Verification items for the finished model (mm, model axes). A direction names the side the tool comes from. Give positions to 0.01 mm unless a question says otherwise; leave off trailing zeros. Loops run counter-clockwise (first coordinate to the right, second up) from the corner with the lowest first, then second, coordinate; pieces in that order, holes last. Notation, with made-up numbers: (-2.5, 42) - (7.5, 42) arc R26 cw to (7.5, 61) - close; hole circle Ø10 at (48.5, -32.75). An arc over 180 degrees is marked (long way). One line per item, written item: value. Start each with the question number.
1. Sectioned sample at C-C (z = 7). Record the cut outline in (x, y), plus the area to 3 significant figures.
2. Mould release check, pull along X, two halves, no side actions. Record for faces 1 (the cylindrical face through (28.35, 39.49, 4.93)), 2 (the cylindrical face through (1, 98, 5)), 3 (the flat face through (103.5, 49, 5)), 4 (the cylindrical face through (99.169, 10.526, 5.07)): pulls with the +X half, pulls with the -X half, needs draft (parallel to the pull), parting line crosses it, or undercut.
3. Sectioned sample at B-B (y = 90). Record the cut outline in (x, z), plus the area to 3 significant figures.
4. Scan lines: L1, parallel to Y at x = 6, z = 4; L2, parallel to X at y = 90, z = 7.75; L3, parallel to X at y = 79, z = 9.75. Record each from-to range of solid material in increasing order. Write a range as [from, to].
5. Sectioned sample at D-D (x = 43.5). Record the cut outline in (y, z).
6. Sectioned sample at A-A (y = 50). Record the cut outline in (x, z), plus the area to 3 significant figures.
7. Access from +Z, -Z, +X, -X, +Y, -Y to the whole of each face (thin tool, end or side, straight path). Record for faces 5 (the flat face through (51, 51, 0)), 6 (the cylindrical face through (28.35, 60.51, 4.93)), 7 (the cylindrical face through (74.99, 39.65, 4.93)).
8. Gauge pin test, flat ends, axial feed: pin 1 (2 mm diameter, centred on x = 6, y = 90, fed in from +Z); pin 2 (6 mm diameter, centred on x = 61.5, z = 3, fed in from +Y); pin 3 (5 mm diameter, centred on x = 50.5, z = 7, fed in from -Y). Record the tip position at first contact, or that the pin passes through.
from build123d import *

# Parameters (mm, degrees)
SKETCH_W        = 103.5
SKETCH_H        = 100
PAD_DEPTH       = 10
SKETCH001_W     = 52.5
SKETCH001_H     = 42.5
POCKET_DEPTH    = 10.001
SKETCH002_R     = 1.75
POCKET001_DEPTH = 10.001
FILLET_R        = 5
FILLET001_R     = 10


with BuildPart() as part:
    # Sketch → Pad (new body)
    with BuildSketch(Plane.XY):
        with Locations((51.75, 50)):
            Rectangle(SKETCH_W, SKETCH_H)
    extrude(amount=PAD_DEPTH)

    # Sketch001 (on Face6 of Pad) → Pocket (cut, through all)
    with BuildSketch(Plane.XY.offset(10)):
        with Locations((51.75, 78.75)):
            Rectangle(SKETCH001_W, SKETCH001_H)
        with Locations((51.75, 21.25)):
            Rectangle(SKETCH001_W, SKETCH001_H)
    extrude(amount=-POCKET_DEPTH, mode=Mode.SUBTRACT)

    # Sketch002 (on Face4 of Pocket) → Pocket001 (cut, through all)
    with BuildSketch(Plane.XY.offset(10)):
        with Locations((6, 90)):
            Circle(SKETCH002_R)
        with Locations((6, 10)):
            Circle(SKETCH002_R)
        with Locations((43.5, 50)):
            Circle(SKETCH002_R)
        with Locations((97.5, 90)):
            Circle(SKETCH002_R)
        with Locations((97.5, 10)):
            Circle(SKETCH002_R)
        with Locations((60, 50)):
            Circle(SKETCH002_R)
    extrude(amount=-POCKET001_DEPTH, mode=Mode.SUBTRACT)

    # Fillet
    fillet_edges = [part.edges().sort_by_distance(p)[0] for p in [
        (0, 100, 5),
        (0, 0, 5),
        (103.5, 0, 5),
        (103.5, 100, 5),
    ]]
    fillet(fillet_edges, radius=FILLET_R)

    # Fillet001
    fillet001_edges = [part.edges().sort_by_distance(p)[0] for p in [
        (78, 57.5, 5),
        (25.5, 42.5, 5),
        (25.5, 57.5, 5),
        (78, 42.5, 5),
    ]]
    fillet(fillet001_edges, radius=FILLET001_R)


solid = part.part
Results are:
1. outline: (0, 5) arc R5 ccw to (5, 0) - (25.5, 0) - (25.5, 32.5) arc R10 cw to (35.5, 42.5) - (68, 42.5) arc R10 cw to (78, 32.5) - (78, 0) - (98.5, 0) arc R5 ccw to (103.5, 5) - (103.5, 95) arc R5 ccw to (98.5, 100) - (78, 100) - (78, 67.5) arc R10 cw to (68, 57.5) - (35.5, 57.5) arc R10 cw to (25.5, 67.5) - (25.5, 100) - (5, 100) arc R5 ccw to (0, 95) - close; hole circle Ø3.5 at (6, 10); hole circle Ø3.5 at (6, 90); hole circle Ø3.5 at (43.5, 50); hole circle Ø3.5 at (60, 50); hole circle Ø3.5 at (97.5, 10); hole circle Ø3.5 at (97.5, 90)
1. area: 5,890 mm^2
2. face 1: undercut
2. face 2: pulls with the -X half
2. face 3: pulls with the +X half
2. face 4: undercut
3. outline: (0, 0) - (4.25, 0) - (4.25, 10) - (0, 10) - close; (7.75, 0) - (25.5, 0) - (25.5, 10) - (7.75, 10) - close; (78, 0) - (95.75, 0) - (95.75, 10) - (78, 10) - close; (99.25, 0) - (103.5, 0) - (103.5, 10) - (99.25, 10) - close
3. area: 440 mm^2
4. L1: y = [0, 8.25], [11.75, 88.25], [91.75, 100]
4. L2: x = [0, 4.25], [7.75, 25.5], [78, 95.75], [99.25, 103.5]
4. L3: x = [0, 25.5], [78, 103.5]
5. outline: (42.5, 0) - (48.25, 0) - (48.25, 10) - (42.5, 10) - close; (51.75, 0) - (57.5, 0) - (57.5, 10) - (51.75, 10) - close
6. outline: (0, 0) - (41.75, 0) - (41.75, 10) - (0, 10) - close; (45.25, 0) - (58.25, 0) - (58.25, 10) - (45.25, 10) - close; (61.75, 0) - (103.5, 0) - (103.5, 10) - (61.75, 10) - close
6. area: 965 mm^2
7. face 5: -Z, +X, -X, +Y, -Y
7. face 6: +Z, -Z, +Y
7. face 7: +Z, -Z, -Y
8. pin 1: passes through
8. pin 2: stops at y = 57.5
8. pin 3: stops at y = 42.5
